```python
from build123d import *

# Parameters (mm, degrees)
F0_R             = 8
F1_DEPTH         = 6
F3_DEPTH         = 2
F4_R             = 2
F5_DEPTH         = 1
F6_R             = 5.5
F7_DEPTH         = 22
F8_R             = 6.5
F8_R_2           = 5.5
F9_DEPTH         = 10
F10_SIZE         = 1
F11_W            = 1
F11_H            = 2
F12_DEPTH        = 20
F12_COPIES_COUNT = 18


# Not quite as in the source:
# - a pattern or mirror of a feature is missing from the dataset's text; its kind, count and spacing are read off the source's solid


with BuildPart() as f1:
    # F0 (on Front) → F1 (new body)
    with BuildSketch(Plane.XZ):
        Circle(F0_R)
    extrude(amount=-F1_DEPTH)

    # F2 (on face) → F3 (join)
    with BuildSketch(Plane.XZ):
        Polygon((1.7320508076, -3), (3.4641016151, 0), (1.7320508076, 3), (-1.7320508076, 3), (-3.4641016151, 0), (-1.7320508076, -3), align=None)
    extrude(amount=F3_DEPTH)

    # F4 (on face) → F5 (join)
    with BuildSketch(Plane.XZ.offset(2)):
        Circle(F4_R)
    extrude(amount=F5_DEPTH)

    # F6 (on face) → F7 (join)
    with BuildSketch(Plane(origin=(0, 6, 0), x_dir=(-1, 0, 0), z_dir=(0, 1, 0))):
        Circle(F6_R)
    extrude(amount=F7_DEPTH)

    # F8 (on face) → F9 (join)
    with BuildSketch(Plane(origin=(0, 28, 0), x_dir=(-1, 0, 0), z_dir=(0, 1, 0))):
        Circle(F8_R)
        Circle(F8_R_2, mode=Mode.SUBTRACT)
    extrude(amount=-F9_DEPTH)

    # F10
    f10_edges = [f1.edges().sort_by_distance(p)[0] for p in [
        (6.5, 28, 0),
    ]]
    chamfer(f10_edges, length=F10_SIZE)

    # F11 (on face) → F12 (cut)
    with BuildSketch(Plane(origin=(0, 28, 0), x_dir=(-1, 0, 0), z_dir=(0, 1, 0))):
        with Locations((0, 6.7)):
            Rectangle(F11_W, F11_H)
    f12 = extrude(amount=-F12_DEPTH, mode=Mode.SUBTRACT)

    # F12_copies: F12 ×18 about axis
    f12_copies_axis = Axis((0, 0, 0), (0, 1, 0))
    for i in range(1, F12_COPIES_COUNT):
        add(f12.rotate(f12_copies_axis, i * 360 / F12_COPIES_COUNT), mode=Mode.SUBTRACT)


solid = f1.part
```
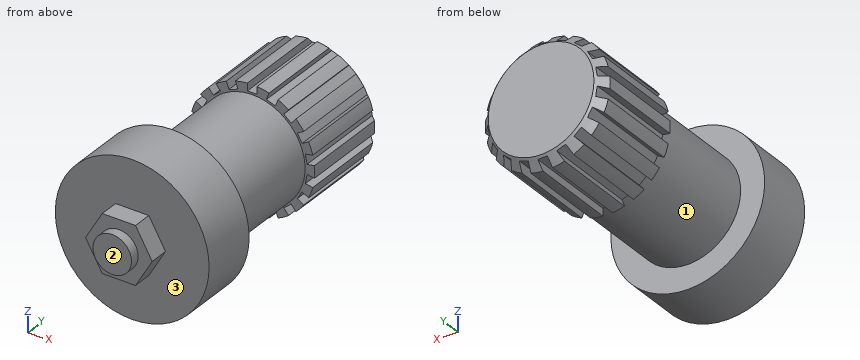
Work out the finished part from the listing and answer in its coordinate system (mm). Face numbers are marked on the shaded views. A direction names the side the tool comes from. Coordinates: 2 decimals unless noted, no trailing zeros. Loops run counter-clockwise (first coordinate to the right, second up) from the corner with the lowest first, then second, coordinate; pieces in that order, holes last. Notation, with made-up numbers: (38.25, 43.5) - (63.25, 43.5) arc R8 cw to (63.25, 57.5) - close; hole circle Ø10 at (-21.75, 60). An arc over 180 degrees is marked (long way). Use a Markdown table: item, result.
Item 1: Given pin 1 Ø1 at (y, z) = (24.5, 2.5) entering from +X; pin 2 Ø0.8 at (x, y) = (0, 25) entering from +Z; pin 3 Ø1 at (y, z) = (3.5, 1.5) entering from -X, each flat-ended and moving along its own axis, determine where each tip first touches the part or whether it passes through.
Evaluation:
| item | result |
|---|---|
| pin 1 | stops at x = 6.18 |
| pin 2 | stops at z = 5.7 |
| pin 3 | stops at x = -7.94 |
Item 2: Find section A-A, the plane x = 0. Determine the outline of the cut face in (y, z).
Evaluation:
| item | result |
|---|---|
| outline | (-3, -2) - (-2, -2) - (-2, -3) - (0, -3) - (0, -8) - (6, -8) - (6, -5.5) - (18, -5.5) - (18, -5.7) - (27.8, -5.7) - (28, -5.5) - (28, 5.5) - (27.8, 5.7) - (18, 5.7) - (18, 5.5) - (6, 5.5) - (6, 8) - (0, 8) - (0, 3) - (-2, 3) - (-2, 2) - (-3, 2) - close |
Item 3: Find section B-B, the plane y = 4.5. Determine the outline of the cut face in (x, z).
Evaluation:
| item | result |
|---|---|
| outline | circle Ø16 at (0, 0) |
Item 4: For the marked faces 1, 2 and 3, determine the directions among +Z, -Z, +X, -X, +Y, -Y from which every point of the face is accessible in a straight line to the end or side of a thin tool.
Evaluation:
| item | result |
|---|---|
| face 1 | none |
| face 2 | +Z, -Z, +X, -X, -Y |
| face 3 | -Y |
Item 5: Consider probe 1 along Y at (x, z) = (2, -1); probe 2 along Y at (x, z) = (-3.5, 4.75); probe 3 along X at (y, z) = (19, -4.25). Determine where each line is inside the solid, lowest interval first. Write a range as from..to.
Evaluation:
| item | result |
|---|---|
| probe 1 | y = -2..28 |
| probe 2 | y = 0..6 |
| probe 3 | x = -4.92..-4.22, -3.8..3.8, 4.22..4.92 |
Item 6: Find section C-C, the plane y = 8.5. Determine the outline of the cut face in (x, z), and give its area (3 significant figures).
Evaluation:
| item | result |
|---|---|
| outline | circle Ø11 at (0, 0) |
| area | 95.0 mm2 |
